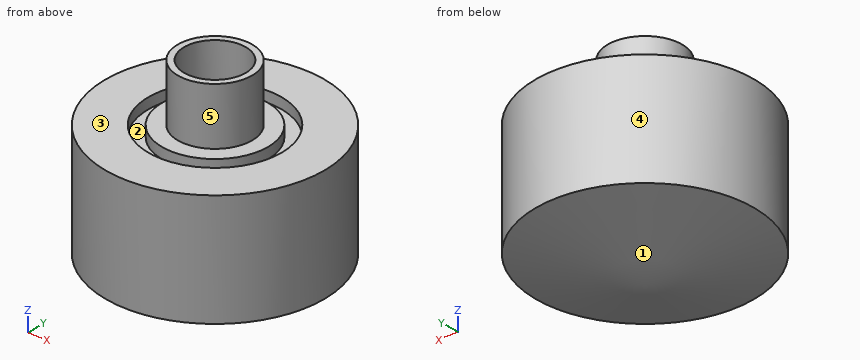
```python
from build123d import *

# Parameters (mm, degrees)
F2_R      = 6.960541
F2_R_2    = 4.7625
F3_DEPTH  = 9.525
F3_FACE_R = 4.7625
F4_DEPTH  = 19.05


with BuildPart() as f1:
    # F0 (on Front) → F1 (revolve)
    with BuildSketch(Plane.XZ):
        Polygon((0, 44.39796), (0, 0), (24.639201, 6.170073), (24.639201, 31.570073), (15.024917, 31.570073), (15.024917, 29.15796), (11.938, 29.15796), (11.938, 31.570073), (8.382, 31.570073), (8.382, 44.39796), align=None)
    revolve(axis=Axis((0, 0, 22.19898), (0, 0, -1)))

    # F2 (on face) → F3 (cut)
    with BuildSketch(Plane.XY.offset(44.39796)):
        Circle(F2_R)
        Circle(F2_R_2, mode=Mode.SUBTRACT)
    extrude(amount=-F3_DEPTH, mode=Mode.SUBTRACT)

    # F3_face (on face) → F4 (cut)
    with BuildSketch(Plane.XY.offset(44.39796)):
        Circle(F3_FACE_R)
    extrude(amount=-F4_DEPTH, mode=Mode.SUBTRACT)


solid = f1.part
```
Read the model definition and answer for the solid it produces. Units are mm, in the model's axes. Face numbers are marked on the shaded views. A direction names the side the tool comes from. Round coordinates to 2 decimals unless told otherwise and drop trailing zeros. Write each loop counter-clockwise with the first axis right and the second up, starting at its lowest first coordinate (ties: lowest second). Pieces come first, ordered by that corner, then holes. Notation, with made-up numbers: (66, -23) - (122, -23) arc R21 ccw to (122, -9) - close; hole circle Ø7 at (3.5, 13). An arc over 180 degrees is marked (long way). One line per item, written item: value.
Q1. For a pull along Y with two mould halves and no side action, classify the marked faces 1, 2 and 3 as pulls with the +Y half, pulls with the -Y half, needs draft (parallel to the pull), parting line crosses it, or undercut.
The answers:
face 1: parting line crosses it
face 2: undercut
face 3: needs draft
Q2. Which of the six approach directions +Z, -Z, +X, -X, +Y, -Y give full straight-line access (tool end or side, diameter ignored) to the marked faces 4 and 5?
The answers:
face 4: +Z, -Z
face 5: +Z
Q3. Find section B-B (z = 12). Determine the outline of the cut face in (x, y).
The answers:
outline: circle Ø49.28 at (0, 0)
Q4. Find section A-A (z = 40). Determine the outline of the cut face in (x, y), and give its area (3 significant figures).
The answers:
outline: circle Ø16.76 at (0, 0); hole circle Ø13.92 at (0, 0)
area: 68.5 mm2
Q5. Straight lines are drawn through the part: line 1 (X direction, y = 1, z = 38); line 2 (X direction, y = -8, z = 29); line 3 (Z direction, x = -0.5, y = -1). For each, find the intervals that lie inside material, in ascending order. Write a range as from..to.
The answers:
line 1: x = -8.32..-6.89, 6.89..8.32
line 2: x = -23.3..23.3
line 3: z = 0.28..25.35
Q6. Each of these flat-tipped pins is pushed along its axis until it touches: P1, Ø7.5, axis at x = 1, y = 0.5, coming from the +Z side; P2, Ø8, axis at y = 16, z = 5.5, coming from the -X side; P3, Ø1, axis at y = 16, z = 14, coming from the -X side. Where does it stop, or does it pass through?
The answers:
P1: stops at z = 34.87
P2: stops at x = -21.49
P3: stops at x = -19.15
Q7. Find section C-C (z = 5.5). Determine the outline of the cut face in (x, y).
The answers:
outline: circle Ø43.93 at (0, 0)
